Autodesk Inventor part; units mm, degrees
ref_plane "YZ Plane" through (0, 0, 0) normal (1, 0, 0) x (0, 1, 0)
ref_plane "XZ Plane" through (0, 0, 0) normal (0, 1, 0) x (-1, 0, 0)
ref_plane "XY Plane" through (0, 0, 0) normal (0, 0, 1) x (1, 0, 0)
sketch "スケッチ1" plane through (0, 0, 0) normal (0, 0, 1) x (1, 0, 0)
  line L0 (44.4, 25) -> (-44.4, 25)
  line L1 (-44.4, 25) -> (-44.4, -25)
  line L2 (-44.4, -25) -> (44.4, -25)
  line L3 (44.4, -25) -> (44.4, 25)
  line L4 (44.4, 25) -> (-44.4, -25) construction
  line L5 (-44.4, 25) -> (44.4, -25) construction
  point P0 (0, 0)
  dimension "d0" = 50
  dimension "d1" = 88.8
extrude "プレート1" add sketch "スケッチ1" along normal mid plane 2
sketch "スケッチ6" plane through (0, 0, -1) normal (0, 0, -1) x (-1, 0, 0)
  circle A0 centre (0, 0) radius 34
  dimension "d48" = 68
extrude "押し出し2" add sketch "スケッチ6" against normal up to surface (2 mm away)
sketch "スケッチ2" plane through (42.4, 25, -1) normal (1, 0, 0) x (0, 1, 0)
  line L0 (-50, 0) -> (0, 0)
  line L1 (0, 0) -> (0, 55)
  line L2 (0, 55) -> (-50, 55)
  line L3 (-50, 55) -> (-50, 0)
edge flange "フランジ1" height 55 angle 90 thickness 2 bend radius 2 thickness toward (1, 0, 0) relief tear relief width 2 relief depth 1 corner gap 2 corner form 0 edges at (44.4, 0, 1) (-44.4, 0, 1) wall of the first edge with corners at (42.4, -25, -1) (42.4, 25, -1) (42.4, 25, 54) (42.4, -25, 54)
bend "曲げ1"
corner "コーナー1"
fillet "フィレット1" radius 25 4 edges at (43.4, 25, 54) (-43.4, 25, 54) (-43.4, -25, 54) (43.4, -25, 54)
sketch "スケッチ3" plane through (44.4, -25, 3) normal (1, 0, 0) x (0, 0, -1)
  arc A0 (-26, 50) -> (-26, 0) centre (-26, 25) ccw
  point P0 (3, 25)
  point P1 (-26, 25)
  point P2 (-38, 25)
  point P3 (-26, 13)
  point P4 (-14, 25)
  point P5 (-26, 37)
  dimension "d24" = 360
  dimension "d52" = 12
hole "穴1" at (44.4, 0, 29) direction (-1, 0, 0) diameter 16 end through all
sketch "スケッチ4" plane through (0, 0, -1) normal (0, 0, -1) x (-1, 0, 0)
  circle A0 centre (0, 0) radius 24
  dimension "d33" = 48
extrude "押し出し1" cut sketch "スケッチ4" against normal through all
sketch "スケッチ5" plane through (0, 0, -1) normal (0, 0, -1) x (-1, 0, 0)
  point P0 (0, 0)
  point P1 (-30, 0)
  point P2 (-15, -25.9808)
  point P3 (15, -25.9808)
  point P4 (30, 0)
  point P5 (15, 25.9808)
  point P6 (-15, 25.9808)
  dimension "d36" = 30
  dimension "d39" = 360
hole "穴3" at (30, 0, -1) at (15, -25.9808, -1) at (-15, -25.9808, -1) at (-30, 0, -1) at (-15, 25.9808, -1) at (15, 25.9808, -1) direction (0, 0, 1) diameter 2.459 end through all
fillet "コーナーR1" radius 12 4 edges at (23.0434, 25, 0) (-23.0434, 25, 0) (23.0434, -25, 0) (-23.0434, -25, 0)
equation "\"d13\" = 0.5 * d0"
equation "\"d46\" = Thickness"
equation "\"d2\" = Thickness"
equation "\"d3\" = BendReliefWidth"
equation "\"d4\" = BendReliefDepth"
equation "\"d5\" = MinimumRemnant"
equation "\"d6\" = TransitionRadius"
equation "\"d9\" = BendRadius"
equation "\"d10\" = CornerReliefSize"
equation "\"d11\" = GapSize"
equation "\"d12\" = JacobiRadiusSize"
equation "\"BendRadius\" = Thickness"
equation "\"BendReliefWidth\" = Thickness"
equation "\"BendReliefDepth\" = 0.5 * Thickness"
equation "\"CornerReliefSize\" = 4 * Thickness"
equation "\"MinimumRemnant\" = 2 * Thickness"
equation "\"TransitionRadius\" = BendRadius"
equation "\"JacobiRadiusSize\" = BendRadius"
equation "\"GapSize\" = Thickness"
properties part number "edge_j4-5" material "アルミニウム 6061"
CAD build for the part. Positions are in the model's coordinates, mm. A direction names the side the tool comes from. Round coordinates to 2 decimals unless told otherwise and drop trailing zeros. Loops run counter-clockwise (first coordinate to the right, second up) from the corner with the lowest first, then second, coordinate; pieces in that order, holes last. Notation, with made-up numbers: M 9,0.5 L 34,0.5 A27 ccw 34,33.5 Z; hole C 18.25,-28.75 d8. An arc over 180 degrees is marked long. Return JSON: item names as keys, results as strings. Group by question number.
(1) Saw through at B-B, the plane x = -30. List the corners of the cut face in (y, z).
(2) Saw through at C-C, the plane y = -14. List the corners of the cut face in (x, z).
(3) Tool access for faces 4 (the cylindrical face through (43, 0, 37)), 5 (the flat face through (19, 16, 1)), 6 (the flat face through (-43, -25, 9)), 7 (the flat face through (43, 25, 9)): list every direction of +Z, -Z, +X, -X, +Y, -Y with a clear straight run to the whole face (end or side of a thin tool).
(4) Wall check: probe 1 along X at (y, z) = (18, 24); probe 2 along Y at (x, z) = (30, 0.2); probe 3 along Y at (x, z) = (-15, 0.3) (3 decimals). Give the ranges that are in metal, low to high. Write a range as [from, to].
(5) Saw through at A-A, the plane z = 15. List the corners of the cut face in (x, y).
(6) Drop flat-ended pins along their axis: P1, Ø19, axis at x = 39.5, z = 8.5, coming from the +Y side; P2, Ø3, axis at x = -15, y = -25.98, coming from the -Z side; P3, Ø2, axis at x = 30, y = 0, coming from the +Z side; P4, Ø4, axis at x = 15, y = 25.98, coming from the +Z side. Give the stop position or say it passes through.
(7) Mould opens along Y. For faces 1 (the flat face through (-44.4, -6, 23)), 2 (the cylindrical face through (-43.414, 17.482, 46.871)), 3 (the cylindrical face through (14.631, 27.154, 0.014)) say: +Y half, -Y half, draft (parallel to the pull), parting line (faces both ways), or undercut.
(8) Saw through at D-D, the plane x = 15. List the corners of the cut face in (y, z) (3 decimals).
Answer list:
{
 "1": {"outline": "M -25,-1 L -1.23,-1 L -1.23,1 L -25,1 Z; M 1.23,-1 L 25,-1 L 25,1 L 1.23,1 Z"},
 "2": {"outline": "M -44.4,3 A4 ccw -40.4,-1 L -19.49,-1 L -19.49,1 L -40.4,1 A2 cw -42.4,3 L -42.4,49.71 L -44.4,49.71 Z; M 19.49,-1 L 40.4,-1 A4 ccw 44.4,3 L 44.4,49.71 L 42.4,49.71 L 42.4,3 A2 cw 40.4,1 L 19.49,1 Z"},
 "3": {"face 4": "+X, -X", "face 5": "+Z, +Y, -Y", "face 6": "+Z, -Z, -X, -Y", "face 7": "+Z, -Z, +X, +Y"},
 "4": {"probe 1": "[-44.4, -42.4], [42.4, 44.4]", "probe 2": "[-25, -1.23], [1.23, 25]", "probe 3": "[-30.512, -27.21], [-24.751, -18.735], [18.735, 24.751], [27.21, 30.512]"},
 "5": {"outline": "M -44.4,-25 L -42.4,-25 L -42.4,25 L -44.4,25 Z; M 42.4,-25 L 44.4,-25 L 44.4,25 L 42.4,25 Z"},
 "6": {"P1": "y = 25", "P2": "z = -1", "P3": "through", "P4": "z = 1"},
 "7": {"face 1": "draft", "face 2": "+Y half", "face 3": "undercut"},
 "8": {"outline": "M -30.512,-1 L -27.21,-1 L -27.21,1 L -30.512,1 Z; M -24.751,-1 L -18.735,-1 L -18.735,1 L -24.751,1 Z; M 18.735,-1 L 24.751,-1 L 24.751,1 L 18.735,1 Z; M 27.21,-1 L 30.512,-1 L 30.512,1 L 27.21,1 Z"}
}
